Source: CAD feature listing. Evaluate the final solid. Frame: model axes, mm. A direction names the side the tool comes from. Give positions to 0.01 mm unless a question says otherwise; leave off trailing zeros. Order: outer loops, then holes, each group sorted by start corner. A loop starts at its lowest first (then second) coordinate and runs counter-clockwise, first axis right, second up. Notation, with made-up numbers: M 70,2 L 110,2 A15 cw 110,10 Z; hole C 47,-13 d9. An arc over 180 degrees is marked long. Answer as a JSON object with one key per item and string values. Group by question number.
1. Section query C-C (y = 3.5). Output: boundary loops of the cut face in (x, z).
2. Pull-direction query (Z, two-part tool) for faces 1 (the cylindrical face through (14.1, 4.06, 15.53)), 2 (the flat face through (2, 6, -2)), 3 (the flat face through (-19, 4, 19)), 4 (the cylindrical face through (2.38, 8.99, -10.74)); classes: +Z half, -Z half, draft (parallel to the pull), parting line (faces both ways), or undercut.
3. Section query B-B (x = 15.6). Output: boundary loops of the cut face in (y, z), plus the area to 3 significant figures.
4. Material intervals for L1, parallel to Z at x = -15.6, y = 4; L2, parallel to Z at x = 15, y = 4, sorted ascending. Write a range as [from, to].
5. Set-up query: faces 5 (the cylindrical face through (-0.867, 8.028, 3.905)), 6 (the cylindrical face through (-16.71, 4.06, 14.59)). Return all of +Z, -Z, +X, -X, +Y, -Y with unobstructed straight access to the full face (end or side cutting, diameter ignored); none if empty.
6. Section query D-D (z = 0). Output: boundary loops of the cut face in (x, y), plus the area to 3 significant figures.
7. Section query A-A (z = -15.6). Output: boundary loops of the cut face in (x, y), plus the area to 3 significant figures.
8. Pin query (flat end, axial travel): P1, Ø2.5, axis at x = -15.6, z = 15.6, coming from the +Y side; P2, Ø10, axis at y = 16, z = 2, coming from the -X side; P3, Ø5, axis at x = 10.5, z = 9.5, coming from the +Y side; P4, Ø1, axis at y = 15.5, z = -0.5, coming from the +X side. Return the tip coordinate at first contact, or that it passes through.
from build123d import *

# Parameters (mm, degrees)
SKETCH1_W               = 42
SKETCH1_H               = 42
BOSS_EXTRUDE1_DEPTH     = 8
SKETCH2_R               = 11
BOSS_EXTRUDE2_DEPTH     = 2
SKETCH3_R               = 4
CUT_EXTRUDE1_DEPTH      = 4
SKETCH4_R               = 2.5
BOSS_EXTRUDE3_DEPTH     = 27
CHAMFER1_SIZE           = 4
SKETCH5_R               = 1.5
CUT_EXTRUDE2_DEPTH      = 26
CUT_EXTRUDE2_DEPTH_BACK = 9


with BuildPart() as part:
    # Sketch1 → Boss-Extrude1 (new body)
    with BuildSketch(Plane(origin=(0, 0, 0), x_dir=(1, 0, 0), z_dir=(0, 1, 0))):
        Rectangle(SKETCH1_W, SKETCH1_H)
    extrude(amount=BOSS_EXTRUDE1_DEPTH)

    # Sketch2 → Boss-Extrude2 (add)
    with BuildSketch(Plane(origin=(0, 8, 0), x_dir=(-1, 0, 0), z_dir=(0, 1, 0))):
        Circle(SKETCH2_R)
    extrude(amount=BOSS_EXTRUDE2_DEPTH)

    # Sketch3 → Cut-Extrude1 (cut)
    with BuildSketch(Plane(origin=(0, 10, 0), x_dir=(1, 0, 0), z_dir=(0, 1, 0))):
        Circle(SKETCH3_R)
    extrude(amount=-CUT_EXTRUDE1_DEPTH, mode=Mode.SUBTRACT)

    # Sketch4 → Boss-Extrude3 (add)
    with BuildSketch(Plane(origin=(0, 6, 0), x_dir=(1, 0, 0), z_dir=(0, 1, 0))):
        Circle(SKETCH4_R)
    extrude(amount=BOSS_EXTRUDE3_DEPTH)

    # Chamfer1
    chamfer1_edges = [part.edges().sort_by_distance(p)[0] for p in [
        (-21, 4, -21),
        (21, 4, -21),
        (21, 4, 21),
        (-21, 4, 21),
    ]]
    chamfer(chamfer1_edges, length=CHAMFER1_SIZE)

    # Sketch5 → Cut-Extrude2 (cut, two sides)
    with BuildSketch(Plane(origin=(0, 8, 0), x_dir=(1, 0, 0), z_dir=(0, 1, 0))) as cut_extrude2_sk:
        with Locations((-15.6, 15.6)):
            Circle(SKETCH5_R)
        with Locations((15.6, 15.6)):
            Circle(SKETCH5_R)
        with Locations((15.6, -15.6)):
            Circle(SKETCH5_R)
        with Locations((-15.6, -15.6)):
            Circle(SKETCH5_R)
    extrude(amount=CUT_EXTRUDE2_DEPTH, mode=Mode.SUBTRACT)
    extrude(cut_extrude2_sk.sketch, amount=-CUT_EXTRUDE2_DEPTH_BACK, mode=Mode.SUBTRACT)


solid = part.part
Answer sheet:
{
 "1": {"outline": "M -21,-17 L -17,-21 L 17,-21 L 21,-17 L 21,17 L 17,21 L -17,21 L -21,17 Z; hole C -15.6,-15.6 d3; hole C -15.6,15.6 d3; hole C 15.6,-15.6 d3; hole C 15.6,15.6 d3"},
 "2": {"face 1": "undercut", "face 2": "undercut", "face 3": "+Z half", "face 4": "parting line"},
 "3": {"outline": "M 0,-21 L 8,-21 L 8,-17.1 L 0,-17.1 Z; M 0,-14.1 L 8,-14.1 L 8,14.1 L 0,14.1 Z; M 0,17.1 L 8,17.1 L 8,21 L 0,21 Z", "area": "288 mm^2"},
 "4": {"L1": "[-21, -17.1], [-14.1, 14.1], [17.1, 21]", "L2": "[-21, -16.97], [-14.23, 14.23], [16.97, 21]"},
 "5": {"face 5": "+Y", "face 6": "+Y, -Y"},
 "6": {"outline": "M -21,0 L 21,0 L 21,8 L 11,8 L 11,10 L 4,10 L 4,6 L 2.5,6 L 2.5,33 L -2.5,33 L -2.5,6 L -4,6 L -4,10 L -11,10 L -11,8 L -21,8 Z", "area": "483 mm^2"},
 "7": {"outline": "M -21,0 L -17.1,0 L -17.1,8 L -21,8 Z; M -14.1,0 L 14.1,0 L 14.1,8 L -14.1,8 Z; M 17.1,0 L 21,0 L 21,8 L 17.1,8 Z", "area": "288 mm^2"},
 "8": {"P1": "through", "P2": "x = -2.5", "P3": "y = 8", "P4": "x = 2.5"}
}
